For this review, take the finished solid that the model builds, in its own axes (mm). A direction names the side the tool comes from. Coordinates: 2 decimals unless noted, no trailing zeros. Loops run counter-clockwise (first coordinate to the right, second up) from the corner with the lowest first, then second, coordinate; pieces in that order, holes last. Notation, with made-up numbers: (-16.75, -34.5) -> (40.25, -34.5) arc R8 cw to (40.25, -29.5) -> close; hole circle Ø10 at (44.5, 9.5). An arc over 180 degrees is marked (long way). Use a Markdown table: item, result.
from build123d import *

# Parameters (mm, degrees)
ESQUISSE1_W        = 140
ESQUISSE1_H        = 42
ESQUISSE1_R        = 5
ESQUISSE1_R_2      = 4
ESQUISSE1_R_3      = 1.5
BOSS_EXTRU_1_DEPTH = 3
CONG_1_R           = 10
CONG_2_R           = 10
ESQUISSE2_R        = 8
ESQUISSE2_R_2      = 4
BOSS_EXTRU_2_DEPTH = 38


with BuildPart() as part:
    # Esquisse1 → Boss.-Extru.1 (new body)
    with BuildSketch(Plane.XY):
        with Locations((-70, 21)):
            Rectangle(ESQUISSE1_W, ESQUISSE1_H)
        with Locations((-70, 32)):
            Circle(ESQUISSE1_R, mode=Mode.SUBTRACT)
        with Locations((-130, 32)):
            Circle(ESQUISSE1_R_2, mode=Mode.SUBTRACT)
        with Locations((-55, 7)):
            Circle(ESQUISSE1_R_3, mode=Mode.SUBTRACT)
        with Locations((-10, 32)):
            Circle(ESQUISSE1_R_2, mode=Mode.SUBTRACT)
        with Locations((-85, 7)):
            Circle(ESQUISSE1_R_3, mode=Mode.SUBTRACT)
    extrude(amount=BOSS_EXTRU_1_DEPTH)

    # Congé1
    cong_1_edges = [part.edges().sort_by_distance(p)[0] for p in [
        (-140, 42, 1.5),
        (0, 42, 1.5),
    ]]
    fillet(cong_1_edges, radius=CONG_1_R)

    # Congé2
    cong_2_edges = [part.edges().sort_by_distance(p)[0] for p in [
        (0, 0, 1.5),
        (-140, 0, 1.5),
    ]]
    fillet(cong_2_edges, radius=CONG_2_R)

    # Esquisse2 → Boss.-Extru.2 (add)
    with BuildSketch(Plane.XY.offset(3)):
        with Locations((-10, 32)):
            Circle(ESQUISSE2_R)
        with Locations((-10, 32)):
            Circle(ESQUISSE2_R_2, mode=Mode.SUBTRACT)
        with Locations((-130, 32)):
            Circle(ESQUISSE2_R)
        with Locations((-130, 32)):
            Circle(ESQUISSE2_R_2, mode=Mode.SUBTRACT)
    extrude(amount=-BOSS_EXTRU_2_DEPTH)


solid = part.part
(1) Take a section at A-A on x = -55. Write out the cut boundary in (y, z).
Found:
| item | result |
|---|---|
| outline | (0, 0) -> (5.5, 0) -> (5.5, 3) -> (0, 3) -> close; (8.5, 0) -> (42, 0) -> (42, 3) -> (8.5, 3) -> close |
(2) For pin 1 Ø7 at (x, y) = (-130, 32) entering from +Z; pin 2 Ø5 at (x, y) = (-97, 5) entering from -Z; pin 3 Ø6 at (y, z) = (25, -15) entering from -X, all flat-tipped, find the tip position at first contact; note any pin that passes through.
Found:
| item | result |
|---|---|
| pin 1 | passes through |
| pin 2 | stops at z = 0 |
| pin 3 | stops at x = -136.93 |
(3) Take a section at B-B on z = -23. Write out the cut boundary in (x, y).
Found:
| item | result |
|---|---|
| outline | circle Ø16 at (-130, 32); circle Ø16 at (-10, 32); hole circle Ø8 at (-130, 32); hole circle Ø8 at (-10, 32) |
(4) For line 1 along Y through (x, z) = (-130, 1); line 2 along Y through (x, z) = (-10, -16.5); line 3 along X through (y, z) = (29, -10.5), list the stretches that pass through material, from the lowest coordinate up.
Found:
| item | result |
|---|---|
| line 1 | y = 0 to 28, 36 to 42 |
| line 2 | y = 24 to 28, 36 to 40 |
| line 3 | x = -137.42 to -132.65, -127.35 to -122.58, -17.42 to -12.65, -7.35 to -2.58 |
(5) Take a section at D-D on x = -70. Write out the cut boundary in (y, z).
Found:
| item | result |
|---|---|
| outline | (0, 0) -> (27, 0) -> (27, 3) -> (0, 3) -> close; (37, 0) -> (42, 0) -> (42, 3) -> (37, 3) -> close |
(6) For faces 1 (the face through (-122.37, 34.4, -17.26)), 2 (the face through (-134, 30, -35)), list the 3-axis set-ups (+Z, -Z, +X, -X, +Y, -Y) from which the entire face can be reached by the end or side of a thin tool; tool diameter is ignored.
Found:
| item | result |
|---|---|
| face 1 | -Z |
| face 2 | -Z, +X, -X, +Y, -Y |
(7) Mouldability with a two-part tool opening along X and no side actions: class faces 3 (the face through (-3.01, 2.85, 1.52)), 4 (the face through (-53.614, 6.425, 1.479)), 5 (the face through (-14, 30, -35)) as pulls with the +X half, pulls with the -X half, needs draft (parallel to the pull), parting line crosses it, or undercut.
Found:
| item | result |
|---|---|
| face 3 | pulls with the +X half |
| face 4 | undercut |
| face 5 | needs draft |
(8) Take a section at C-C on y = 34.5. Write out the cut boundary in (x, z).
Found:
| item | result |
|---|---|
| outline | (-139.68, 0) -> (-137.6, 0) -> (-137.6, -35) -> (-133.12, -35) -> (-133.12, 3) -> (-139.68, 3) -> close; (-126.88, -35) -> (-122.4, -35) -> (-122.4, 0) -> (-74.33, 0) -> (-74.33, 3) -> (-126.88, 3) -> close; (-65.67, 0) -> (-17.6, 0) -> (-17.6, -35) -> (-13.12, -35) -> (-13.12, 3) -> (-65.67, 3) -> close; (-6.88, -35) -> (-2.4, -35) -> (-2.4, 0) -> (-0.32, 0) -> (-0.32, 3) -> (-6.88, 3) -> close |
